Input: dimensioned drawing with shaded views. Units: mm. Origin: part minimum x, y, z. A direction names the side the tool comes from. Give positions to 0.01 mm unless a question says otherwise; leave off trailing zeros. Write each loop counter-clockwise with the first axis right and the second up, starting at its lowest first coordinate (ties: lowest second). Pieces come first, ordered by that corner, then holes.
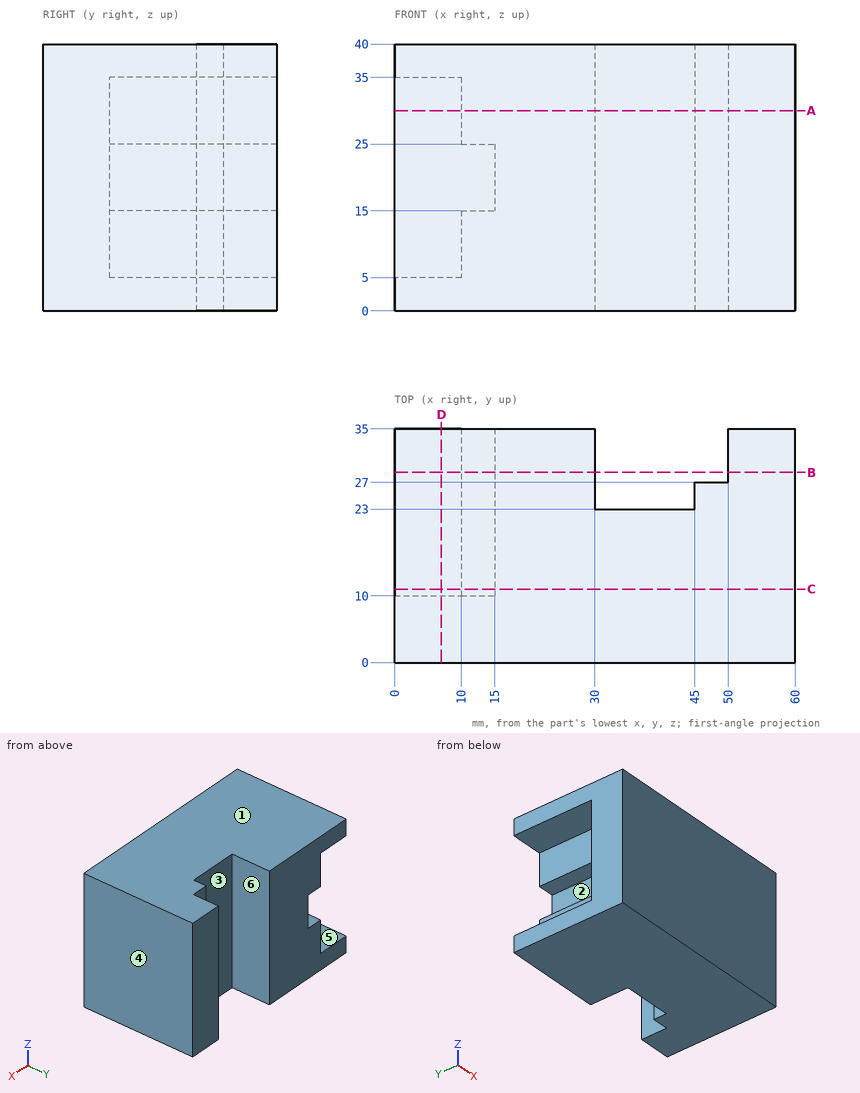
Item 1: Section B-B, the plane y = 28.5. Return the cut outline in (x, z), plus the area to 3 significant figures.
Found:
outline: (0, 0) - (30, 0) - (30, 40) - (0, 40) - (0, 35) - (10, 35) - (10, 25) - (15, 25) - (15, 15) - (10, 15) - (10, 5) - (0, 5) - close; (50, 0) - (60, 0) - (60, 40) - (50, 40) - close
area: 1,250 mm2
Item 2: Section D-D, the plane x = 7. Return the cut outline in (y, z).
Found:
outline: (0, 0) - (35, 0) - (35, 5) - (10, 5) - (10, 35) - (35, 35) - (35, 40) - (0, 40) - close
Item 3: Pin query (flat end, axial travel): pin 1 Ø3 at (y, z) = (28.5, 32) entering from -X; pin 2 Ø10 at (y, z) = (8.5, 16) entering from -X; pin 3 Ø2.5 at (x, z) = (48.5, 19) entering from +Y; pin 4 Ø2.5 at (y, z) = (29, 18) entering from -X. Return the tip coordinate at first contact, or that it passes through.
Found:
pin 1: stops at x = 10
pin 2: stops at x = 0
pin 3: stops at y = 27
pin 4: stops at x = 15
Item 4: Section A-A, the plane z = 30. Return the cut outline in (x, y).
Found:
outline: (0, 0) - (60, 0) - (60, 35) - (50, 35) - (50, 27) - (45, 27) - (45, 23) - (30, 23) - (30, 35) - (10, 35) - (10, 10) - (0, 10) - close
Item 5: Reachability of the marked faces 4, 5 and 6 from +Z, -Z, +X, -X, +Y, -Y: full face, straight path, thin tool, end or side. Return the list, or none.
Found:
face 4: +Z, -Z, +X, +Y, -Y
face 5: -X, +Y
face 6: +Z, -Z, +Y
Item 6: Section C-C, the plane y = 11. Return the cut outline in (x, z), plus the area to 3 significant figures.
Found:
outline: (0, 0) - (60, 0) - (60, 40) - (0, 40) - (0, 35) - (10, 35) - (10, 25) - (15, 25) - (15, 15) - (10, 15) - (10, 5) - (0, 5) - close
area: 2,050 mm2
Item 7: Pull-direction query (Z, two-part tool) for the marked faces 1, 2 and 3; classes: +Z half, -Z half, draft (parallel to the pull), parting line (faces both ways), or undercut.
Found:
face 1: +Z half
face 2: undercut
face 3: draft
Item 8: Line query: L1, parallel to X at y = 24, z = 34.5; L2, parallel to Z at x = 12.5, y = 11; L3, parallel to X at y = 33.5, z = 26. Output: solid intervals per line, ascending.
Found:
L1: x = 10 to 30, 45 to 60
L2: z = 0 to 15, 25 to 40
L3: x = 10 to 30, 50 to 60
